Verification items for this drawing (mm, ordinates from the low corner). Round coordinates to 2 decimals unless told otherwise and drop trailing zeros. Order: outer loops, then holes, each group sorted by start corner. A loop starts at its lowest first (then second) coordinate and runs counter-clockwise, first axis right, second up. Notation, with made-up numbers: (-27.75, 82.5) -> (1.25, 82.5) arc R5 cw to (1.25, 86.5) -> close; hole circle Ø8 at (62.5, 32). An arc over 180 degrees is marked (long way). Answer in a Markdown table with one row per item. Add a question column.
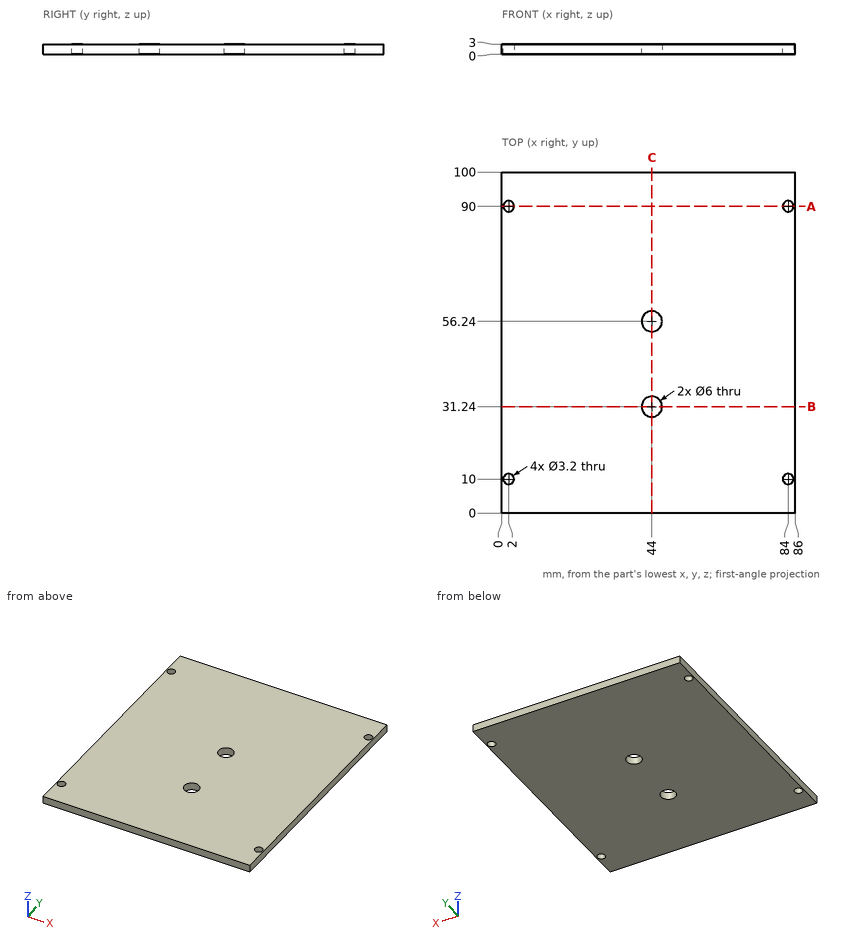
1) Cross-section at B-B, the plane y = 31.24. Record the boundary of the cut face in (x, z).
2) Cross-section at A-A, the plane y = 90. Record the boundary of the cut face in (x, z).
3) Depth check by flat-ended pin: P1, Ø4, axis at x = 2, y = 90, coming from the -Z side. Enter the tip coordinate at first touch or a pass-through.
4) Thickness scan on L1, parallel to Y at x = 2, z = 1.1. Record the ranges inside material, lowest first. Write a range as [from, to].
5) Cross-section at C-C, the plane x = 44. Record the boundary of the cut face in (y, z).
Results below:
| question | item | result |
|---|---|---|
| 1 | outline | (0, 0) -> (41, 0) -> (41, 3) -> (0, 3) -> close; (47, 0) -> (86, 0) -> (86, 3) -> (47, 3) -> close |
| 2 | outline | (0, 0) -> (0.4, 0) -> (0.4, 3) -> (0, 3) -> close; (3.6, 0) -> (82.4, 0) -> (82.4, 3) -> (3.6, 3) -> close; (85.6, 0) -> (86, 0) -> (86, 3) -> (85.6, 3) -> close |
| 3 | P1 | z = 0 |
| 4 | L1 | [0, 8.4], [11.6, 88.4], [91.6, 100] |
| 5 | outline | (0, 0) -> (28.24, 0) -> (28.24, 3) -> (0, 3) -> close; (34.24, 0) -> (53.24, 0) -> (53.24, 3) -> (34.24, 3) -> close; (59.24, 0) -> (100, 0) -> (100, 3) -> (59.24, 3) -> close |
